Verification items for the finished model (mm, model axes). A direction names the side the tool comes from. Coordinates: 2 decimals unless noted, no trailing zeros. Order: outer loops, then holes, each group sorted by start corner. A loop starts at its lowest first (then second) coordinate and runs counter-clockwise, first axis right, second up.
Q1. Cross-section at D-D, the plane y = 6. Record the boundary of the cut face in (x, z).
Q2. Thickness scan on line 1 (X direction, y = 0.25, z = 1.05); line 2 (X direction, y = -4.25, z = 3.3); line 3 (Y direction, x = 1.25, z = 1.05). Record the ranges inside material, lowest first.
Q3. Cross-section at C-C, the plane z = 0.55. Record the boundary of the cut face in (x, y).
Q4. Cross-section at A-A, the plane y = 0. Record the boundary of the cut face in (x, z), and give its area (3 significant figures).
Q5. Cross-section at B-B, the plane x = 0. Record the boundary of the cut face in (y, z).
Q6. Depth check by flat-ended pin: P1, Ø3, axis at y = -6, z = 5.5, coming from the -X side; P2, Ø1.5, axis at x = -3, z = 1.5, coming from the -Y side; P3, Ø1, axis at x = -7, z = 5, coming from the -Y side. Enter the tip coordinate at first touch or a pass-through.
Q7. Draft check along Y on faces 3 (the flat face through (1.5, 0, 3)), 4 (the cylindrical face through (-2.17, -9.76, 2.96)), 5 (the flat face through (2, 0, 0)). Enter one of: pulls with the +Y half, pulls with the -Y half, needs draft (parallel to the pull), parting line crosses it, or undercut.
Q8. Set-up check for faces 1 (the flat face through (2, 0, 6)), 2 (the cylindrical face through (0, 5, 3)): record each of +Z, -Z, +X, -X, +Y, -Y from which the full face is reachable in a straight line by a thin tool's end or side.
from build123d import *

# Parameters (mm, degrees)
F0_R     = 10
F1_DEPTH = 6


with BuildPart() as f1:
    # F0 (on Top) → F1 (new body)
    with BuildSketch(Plane.XY):
        Circle(F0_R)
        with BuildLine():
            ThreePointArc((1.5, 4.7696960071), (4.0311288741, 2.9580398915), (5, 0))
            ThreePointArc((5, 0), (4.0311288741, -2.9580398915), (1.5, -4.7696960071))
            Line((1.5, -4.7696960071), (1.5, -5.7218258735))
            Line((1.5, -5.7218258735), (-1.5, -5.7218258735))
            Line((-1.5, -5.7218258735), (-1.5, -4.7696960071))
            ThreePointArc((-1.5, -4.7696960071), (-5, 0), (-1.5, 4.7696960071))
            Line((-1.5, 4.7696960071), (-1.5, 5.7218258735))
            Line((-1.5, 5.7218258735), (1.5, 5.7218258735))
            Line((1.5, 5.7218258735), (1.5, 4.7696960071))
        make_face(mode=Mode.SUBTRACT)
        with BuildLine():
            Line((-1.5, -4.7696960071), (-1.5, 4.7696960071))
            ThreePointArc((-1.5, 4.7696960071), (-5, 0), (-1.5, -4.7696960071))
        make_face()
        with BuildLine():
            ThreePointArc((1.5, -4.7696960071), (4.0311288741, -2.9580398915), (5, 0))
            ThreePointArc((5, 0), (4.0311288741, 2.9580398915), (1.5, 4.7696960071))
            Line((1.5, 4.7696960071), (1.5, -4.7696960071))
        make_face()
        with BuildLine():
            ThreePointArc((-1.5, 4.7696960071), (0, 5), (1.5, 4.7696960071))
            Line((1.5, 4.7696960071), (1.5, 5.7218258735))
            Line((1.5, 5.7218258735), (-1.5, 5.7218258735))
            Line((-1.5, 5.7218258735), (-1.5, 4.7696960071))
        make_face()
        with BuildLine():
            Line((1.5, -5.7218258735), (1.5, -4.7696960071))
            ThreePointArc((1.5, -4.7696960071), (0, -5), (-1.5, -4.7696960071))
            Line((-1.5, -4.7696960071), (-1.5, -5.7218258735))
            Line((-1.5, -5.7218258735), (1.5, -5.7218258735))
        make_face()
    extrude(amount=F1_DEPTH)


solid = f1.part
Check values:
1. outline: (-8, 0) - (8, 0) - (8, 6) - (-8, 6) - close
2. line 1: x = -10 to -1.5, 1.5 to 10
2. line 2: x = -9.05 to -1.5, 1.5 to 9.05
2. line 3: y = -9.92 to -4.84, 4.84 to 9.92
3. outline: circle Ø20 at (0, 0); hole (-1.5, -4.77) arc R5 ccw to (1.5, -4.77) - (1.5, 4.77) arc R5 ccw to (-1.5, 4.77) - close
4. outline: (-10, 0) - (-1.5, 0) - (-1.5, 6) - (-10, 6) - close; (1.5, 0) - (10, 0) - (10, 6) - (1.5, 6) - close
4. area: 102 mm2
5. outline: (-10, 0) - (-5, 0) - (-5, 6) - (-10, 6) - close; (5, 0) - (10, 0) - (10, 6) - (5, 6) - close
6. P1: stops at x = -8.93
6. P2: stops at y = -9.74
6. P3: stops at y = -7.6
7. face 3: undercut
7. face 4: parting line crosses it
7. face 5: needs draft
8. face 1: +Z, +X, -X, +Y, -Y
8. face 2: +Z, -Z
